from build123d import *

# Parameters (mm, degrees)
F0_W          = 13.3
F0_H          = 13.3
F0_W_2        = 10.3
F0_H_2        = 10.3
F1_DEPTH      = 20
F2_DEPTH      = 1.5
F3_W          = 5
F3_H          = 13.3
F4_DEPTH      = 13.3
F5_T1_DEPTH   = 38.3
F6_R          = 2.55
F7_DEPTH      = 25
F7_DEPTH_BACK = 25


# Not quite as in the source:
# - a fillet or chamfer that OpenCascade refuses, or shapes differently, is made with other operations: its cross-section is extruded or revolved along the edge and cut away or added


with BuildPart() as f1:
    # F0 (on Top) → F1 (new body)
    with BuildSketch(Plane.XY):
        Rectangle(F0_W, F0_H)
        Rectangle(F0_W_2, F0_H_2, mode=Mode.SUBTRACT)
    extrude(amount=-F1_DEPTH)

    # F0 (on Top) → F2 (join)
    with BuildSketch(Plane.XY):
        Rectangle(F0_W, F0_H)
        Rectangle(F0_W_2, F0_H_2, mode=Mode.SUBTRACT)
        Rectangle(F0_W_2, F0_H_2)
    extrude(amount=F2_DEPTH)

    # F3 (on face) → F4 (join)
    with BuildSketch(Plane.XY.offset(1.5)):
        Rectangle(F3_W, F3_H)
    extrude(amount=F4_DEPTH)

    # F5: fillet of radius 6.66 on 2 edges, made by hand

    # F5_s2 → F5_t1 (cut)
    with BuildSketch(Plane.YZ.offset(-19.15)):
        with BuildLine():
            ThreePointArc((-6.65, 8.14), (-4.6993311627, 12.8493311627), (0.01, 14.8))
            Line((0.01, 14.8), (-6.65, 14.8))
            Line((-6.65, 14.8), (-6.65, 8.14))
        make_face()
        with BuildLine():
            ThreePointArc((6.65, 8.14), (4.6993311627, 12.8493311627), (-0.01, 14.8))
            Line((-0.01, 14.8), (6.65, 14.8))
            Line((6.65, 14.8), (6.65, 8.14))
        make_face()
    extrude(amount=F5_T1_DEPTH, mode=Mode.SUBTRACT)

    # F6 (on face) → F7 (cut, two sides)
    with BuildSketch(Plane.YZ.offset(2.5)) as f7_sk:
        with Locations((0, 8.14)):
            Circle(F6_R)
    extrude(amount=-F7_DEPTH, mode=Mode.SUBTRACT)
    extrude(f7_sk.sketch, amount=F7_DEPTH_BACK, mode=Mode.SUBTRACT)


solid = f1.part
Read the model definition and answer for the solid it produces. Units are mm, in the model's axes. A direction names the side the tool comes from. Round coordinates to 2 decimals unless told otherwise and drop trailing zeros. Write each loop counter-clockwise with the first axis right and the second up, starting at its lowest first coordinate (ties: lowest second). Pieces come first, ordered by that corner, then holes. Notation, with made-up numbers: M -27.5,76 L -9.5,76 A19 cw -9.5,113 Z; hole C 70,36 d10. An arc over 180 degrees is marked long. Use a Markdown table: item, result.
1) The part is cut by section B-B (x = -2). Write down the section's boundary in (y, z).
Answers follow:
| item | result |
|---|---|
| outline | M -6.65,-20 L -5.15,-20 L -5.15,0 L 5.15,0 L 5.15,-20 L 6.65,-20 L 6.65,8.14 A6.66 ccw 0,14.8 A6.66 ccw -6.65,8.14 Z; hole C 0,8.14 d5.1 |
2) The part is cut by section A-A (z = -10). Write down the section's boundary in (x, y).
Answers follow:
| item | result |
|---|---|
| outline | M -6.65,-6.65 L 6.65,-6.65 L 6.65,6.65 L -6.65,6.65 Z; hole M -5.15,-5.15 L 5.15,-5.15 L 5.15,5.15 L -5.15,5.15 Z |
3) For a pull along Y with two mould halves and no side action, classify faces 1 (the cylindrical face through (-0.035, 4.754, 12.794)), 2 (the cylindrical face through (0.04, 1.18, 5.88)), 3 (the flat face through (-6.65, 0, -9)) as pulls with the +Y half, pulls with the -Y half, needs draft (parallel to the pull), parting line crosses it, or undercut.
Answers follow:
| item | result |
|---|---|
| face 1 | pulls with the +Y half |
| face 2 | undercut |
| face 3 | needs draft |
4) Straight lines are drawn through the part: line 1 along Z through (x, y) = (1.05, 0); line 2 along Y through (x, z) = (-1.75, -7). For each, find the intervals that lie inside material, in ascending order. Write a range as [from, to].
Answers follow:
| item | result |
|---|---|
| line 1 | z = [0, 5.59], [10.69, 14.8] |
| line 2 | y = [-6.65, -5.15], [5.15, 6.65] |
5) A tool of negligible diameter and unlimited length cuts with its end or side. For faces 4 (the flat face through (2.5, 0, 5)), 5 (the flat face through (0, 5.15, -10)), 6 (the flat face through (-2.5, 0, 5)), 7 (the flat face through (0, -6.65, -9)), from which of +Z, -Z, +X, -X, +Y, -Y can it reach the whole face along a straight path? Write none if from no direction.
Answers follow:
| item | result |
|---|---|
| face 4 | +Z, +X, +Y, -Y |
| face 5 | -Z |
| face 6 | +Z, -X, +Y, -Y |
| face 7 | +Z, -Z, +X, -X, -Y |
6) The part is cut by section D-D (x = -4). Write down the section's boundary in (y, z).
Answers follow:
| item | result |
|---|---|
| outline | M -6.65,-20 L -5.15,-20 L -5.15,0 L 5.15,0 L 5.15,-20 L 6.65,-20 L 6.65,1.5 L -6.65,1.5 Z |
7) Flat-ended cylindrical pins translate along their axes: pin 1 (4 mm diameter, centred on y = 2.5, z = 8, fed in from -X); pin 2 (3.5 mm diameter, centred on x = 4.5, y = -2, fed in from +Z); pin 3 (1.5 mm diameter, centred on x = -4, y = -1.5, fed in from -Z). Find the tip coordinate at first contact, or state that the pin passes through.
Answers follow:
| item | result |
|---|---|
| pin 1 | stops at x = -2.5 |
| pin 2 | stops at z = 1.5 |
| pin 3 | stops at z = 0 |
8) The part is cut by section C-C (y = -1.75). Write down the section's boundary in (x, z).
Answers follow:
| item | result |
|---|---|
| outline | M -6.65,-20 L -5.15,-20 L -5.15,0 L 5.15,0 L 5.15,-20 L 6.65,-20 L 6.65,1.5 L 2.5,1.5 L 2.5,6.29 L -2.5,6.29 L -2.5,1.5 L -6.65,1.5 Z; M -2.5,9.99 L 2.5,9.99 L 2.5,14.56 L -2.5,14.56 Z |
